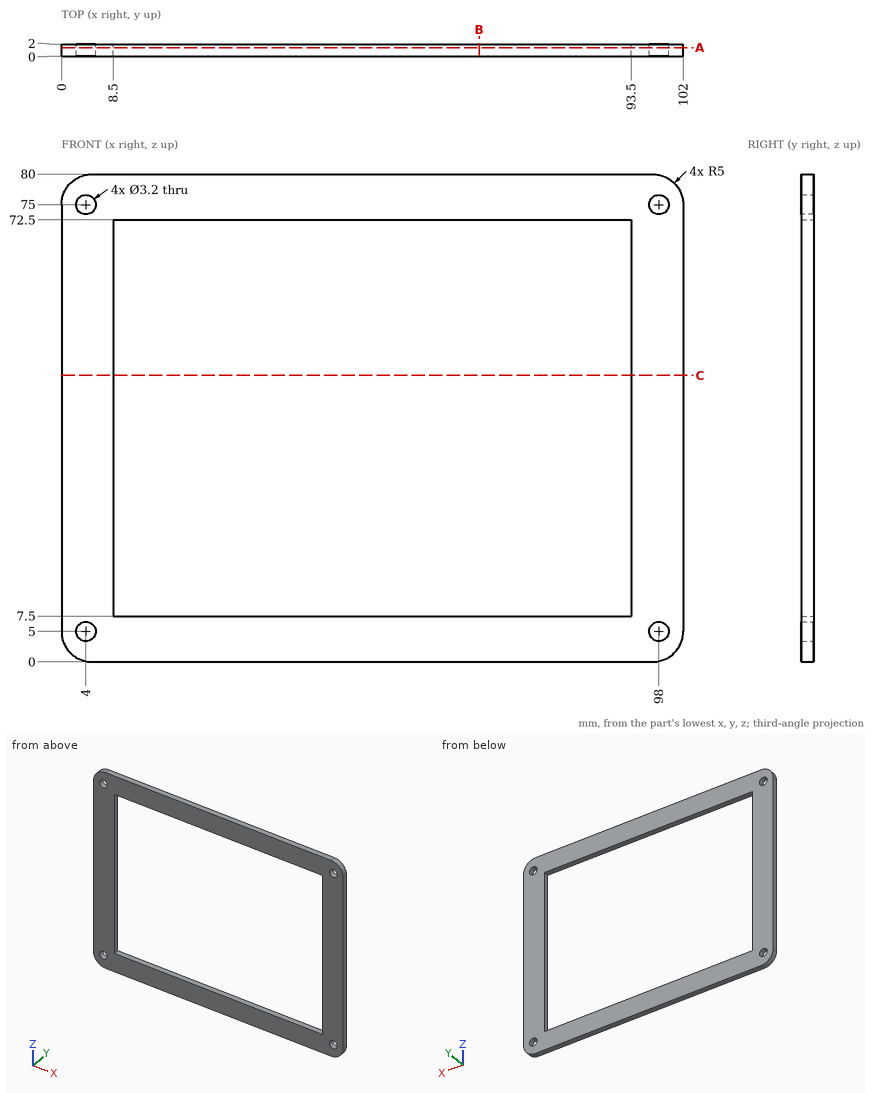
Drawing for the job (mm, zero at the part's lowest x, y, z). Round coordinates to 2 decimals unless told otherwise and drop trailing zeros. Write each loop counter-clockwise with the first axis right and the second up, starting at its lowest first coordinate (ties: lowest second). Pieces come first, ordered by that corner, then holes. Notation, with made-up numbers: (4.25, 32.5) - (59.25, 32.5) arc R7 cw to (59.25, 42.5) - close; hole circle Ø4 at (21.25, -27.75). An arc over 180 degrees is marked (long way). Return JSON: item names as keys, results as strings. Group by question number.
Item 1: Flat gauge pin, fed straight in: pin 1 Ø3.5 at (x, z) = (4, 75) entering from -Y. Where does the tip first touch, or does it go through?
Item 2: Band-saw the part on A-A on y = 1.4. List the corners of the cut face in (x, z).
Item 3: Band-saw the part on C-C on z = 47. List the corners of the cut face in (x, y), plus the area to 3 significant figures.
Item 4: Probe probe 1 along X at (y, z) = (1.4, 5); probe 2 along Z at (x, y) = (22.5, 0.6); probe 3 along X at (y, z) = (1.7, 66). List the from-to ranges inside material, lowest first.
Item 5: Band-saw the part on B-B on x = 68.5. List the corners of the cut face in (y, z).
Resolved:
{
 "1": {"pin 1": "stops at y = 0"},
 "2": {"outline": "(0, 5) arc R5 ccw to (5, 0) - (97, 0) arc R5 ccw to (102, 5) - (102, 75) arc R5 ccw to (97, 80) - (5, 80) arc R5 ccw to (0, 75) - close; hole circle Ø3.2 at (4, 5); hole circle Ø3.2 at (4, 75); hole (8.5, 7.5) - (93.5, 7.5) - (93.5, 72.5) - (8.5, 72.5) - close; hole circle Ø3.2 at (98, 5); hole circle Ø3.2 at (98, 75)"},
 "3": {"outline": "(0, 0) - (8.5, 0) - (8.5, 2) - (0, 2) - close; (93.5, 0) - (102, 0) - (102, 2) - (93.5, 2) - close", "area": "34.0 mm²"},
 "4": {"probe 1": "x = 0 to 2.4, 5.6 to 96.4, 99.6 to 102", "probe 2": "z = 0 to 7.5, 72.5 to 80", "probe 3": "x = 0 to 8.5, 93.5 to 102"},
 "5": {"outline": "(0, 0) - (2, 0) - (2, 7.5) - (0, 7.5) - close; (0, 72.5) - (2, 72.5) - (2, 80) - (0, 80) - close"}
}
